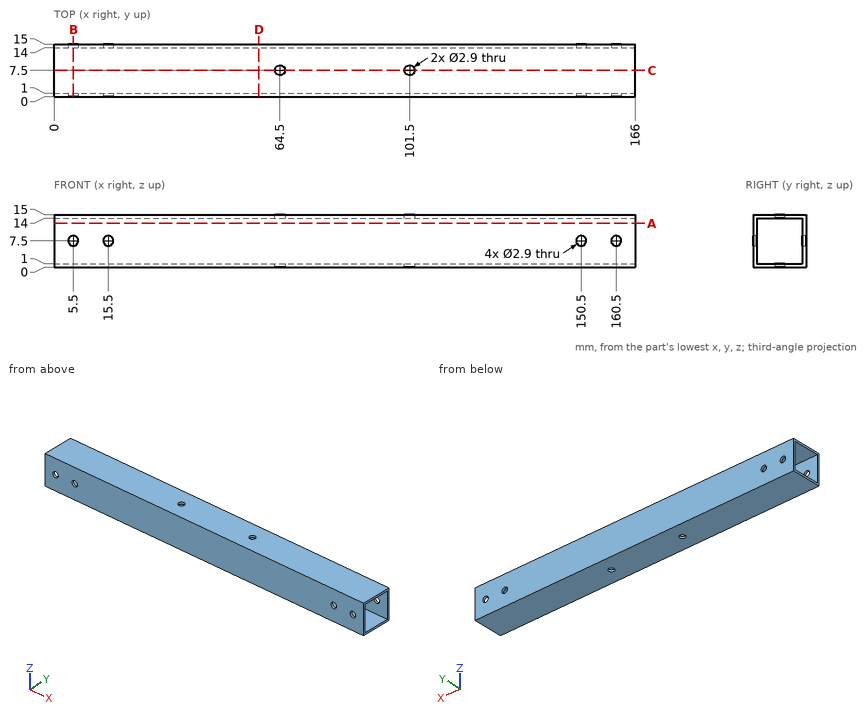
Geometry check sheet. Reference: drawing and pictorial views, mm from the part's lowest x, y, z. Round coordinates to 2 decimals unless told otherwise and drop trailing zeros. Loops run counter-clockwise (first coordinate to the right, second up) from the corner with the lowest first, then second, coordinate; pieces in that order, holes last. Notation, with made-up numbers: M -33,86.25 L 26,86.25 A10 cw 26,99.25 Z; hole C -11.75,30.25 d7. An arc over 180 degrees is marked long. Return JSON: item names as keys, results as strings. Group by question number.
(1) Section check C-C, the plane y = 7.5. Enter the section's corners in (x, z).
(2) Section check A-A, the plane z = 12.5. Enter the section's corners in (x, y), and give its area (3 significant figures).
(3) Section check D-D, the plane x = 58.5. Enter the section's corners in (y, z).
(4) Section check B-B, the plane x = 5.5. Enter the section's corners in (y, z).
(5) Scan lines: line 1 along X through (y, z) = (14.35, 7.5); line 2 along Z through (x, y) = (154, 9.25). Record each from-to range of solid material in increasing order. Write a range as [from, to].
(6) Go/stop test with flat-tipped pins: pin 1 (2.5 mm diameter, centred on x = 5.5, z = 7.5, fed in from -Y); pin 2 (6.5 mm diameter, centred on x = 116.5, y = 5, fed in from -Z). Record where each tip stops, or that it passes through.
Data:
{
 "1": {"outline": "M 0,0 L 63.05,0 L 63.05,1 L 0,1 Z; M 0,14 L 63.05,14 L 63.05,15 L 0,15 Z; M 65.95,0 L 100.05,0 L 100.05,1 L 65.95,1 Z; M 65.95,14 L 100.05,14 L 100.05,15 L 65.95,15 Z; M 102.95,0 L 166,0 L 166,1 L 102.95,1 Z; M 102.95,14 L 166,14 L 166,15 L 102.95,15 Z"},
 "2": {"outline": "M 0,0 L 166,0 L 166,1 L 0,1 Z; M 0,14 L 166,14 L 166,15 L 0,15 Z", "area": "332 mm²"},
 "3": {"outline": "M 0,0 L 15,0 L 15,15 L 0,15 Z; hole M 1,1 L 14,1 L 14,14 L 1,14 Z"},
 "4": {"outline": "M 0,0 L 15,0 L 15,6.05 L 14,6.05 L 14,1 L 1,1 L 1,6.05 L 0,6.05 Z; M 0,8.95 L 1,8.95 L 1,14 L 14,14 L 14,8.95 L 15,8.95 L 15,15 L 0,15 Z"},
 "5": {"line 1": "[0, 4.05], [6.95, 14.05], [16.95, 149.05], [151.95, 159.05], [161.95, 166]", "line 2": "[0, 1], [14, 15]"},
 "6": {"pin 1": "through", "pin 2": "z = 0"}
}
